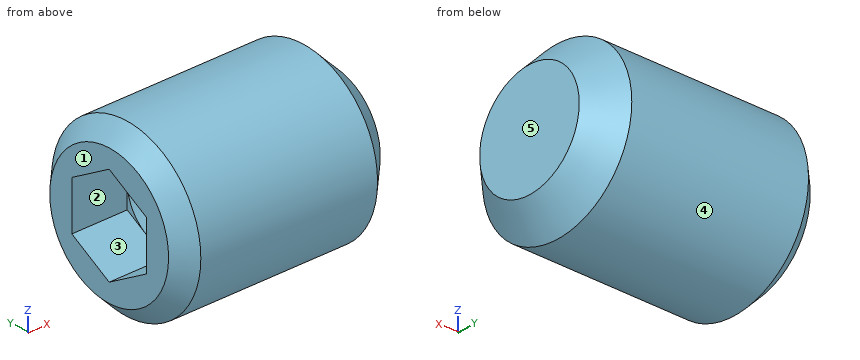
Autodesk Inventor part; units mm, degrees
ref_plane "CP_XY" through (0, 0, 0) normal (1, 0, 0) x (0, 0, -1)
ref_plane "CP_YZ" through (0, 0, 0) normal (0, 0, -1) x (0, 1, 0)
ref_plane "CP_ZX" through (0, 0, 0) normal (0, 1, 0) x (1, 0, 0)
sketch "Sketch_1" plane through (0, 0, 0) normal (0, 0, 1) x (1, 0, 0)
  line L0 (0, 0) -> (-8, 0)
  line L1 (-8, 0) -> (-8, 2.3865)
  line L2 (-8, 2.3865) -> (-7.3865, 3)
  line L3 (-7.3865, 3) -> (-1, 3)
  line L4 (-1, 3) -> (0, 2)
  line L5 (0, 2) -> (0, 0)
  line L6 (0, 0) -> (-8, 0)
revolve "Revolution1" add sketch "Sketch_1" angle 360 about axis through (0, 0, 0) along (1, 0, 0)
thread "Thread1"
sketch "Sketch_2" plane through (-8, 0, 0) normal (-1, 0, 0) x (0, 1, 0)
  line L0 (-1.5, -0.866) -> (0, -1.7321)
  line L1 (0, -1.7321) -> (1.5, -0.866)
  line L2 (1.5, -0.866) -> (1.5, 0.866)
  line L3 (1.5, 0.866) -> (0, 1.7321)
  line L4 (0, 1.7321) -> (-1.5, 0.866)
  line L5 (-1.5, 0.866) -> (-1.5, -0.866)
extrude "Extrusion1" cut sketch "Sketch_2" against normal blind 2
sketch "Sketch_3" plane through (0, 0, 0) normal (0, 0, 1) x (1, 0, 0)
  line L0 (-5.134, 0) -> (-6, 0)
  line L1 (-6, 0) -> (-6, 1.5)
  line L2 (-6, 1.5) -> (-5.134, 0)
  line L3 (-5.134, 0) -> (-6, 0)
revolve "Revolution2" cut sketch "Sketch_3" angle 360 about axis through (-5.134, 0, 0) along (1, 0, 0)
ref_plane "CP_XY" through (0, 0, 0) normal (1, 0, 0) x (0, 0, -1)
ref_plane "CP_YZ" through (0, 0, 0) normal (0, 0, -1) x (0, 1, 0)
ref_plane "CP_ZX" through (0, 0, 0) normal (0, 1, 0) x (1, 0, 0)
properties part number "SET-SCREW6-8"
Source: CAD feature listing. Evaluate the final solid. Frame: model axes, mm. Face numbers are marked on the shaded views. A direction names the side the tool comes from. Round coordinates to 2 decimals unless told otherwise and drop trailing zeros. Write each loop counter-clockwise with the first axis right and the second up, starting at its lowest first coordinate (ties: lowest second). Pieces come first, ordered by that corner, then holes. Notation, with made-up numbers: M -2.5,-10 L 27.5,-10 A15 ccw 27.5,-5 Z; hole C 34,34.5 d4. An arc over 180 degrees is marked long. One line per item, written item: value. Start each with the question number.
Item 1: Section query B-B (x = -1.25). Return the cut outline in (y, z), plus the area to 3 significant figures.
Item 2: Pin query (flat end, axial travel): pin 1 (0.9 mm diameter, centred on y = 0, z = -1, fed in from -X); pin 2 (1 mm diameter, centred on x = -2.5, z = 2, fed in from -Y); pin 3 (0.5 mm diameter, centred on x = -6.5, z = -0.5, fed in from +Y). Return the tip coordinate at first contact, or that it passes through.
Item 3: Mould query, pull axis Z, two halves, no side actions, for the marked faces 3, 4 and 5. Classes: pulls with the +Z half, pulls with the -Z half, needs draft (parallel to the pull), parting line crosses it, or undercut.
Item 4: Section query C-C (x = -5.5). Return the cut outline in (y, z).
Item 5: Set-up query: the marked faces 1 and 2. Return all of +Z, -Z, +X, -X, +Y, -Y with unobstructed straight access to the full face (end or side cutting, diameter ignored); none if empty.
Item 6: Ray query, L1, parallel to Z at x = -7.5, y = -1.3; L2, parallel to Y at x = -1.25, z = -2.45; L3, parallel to Y at x = -6, z = -1.75. Return the intervals inside material, ascending. Write a range as from..to.
Item 7: Section query A-A (x = -7.5). Return the cut outline in (y, z), plus the area to 3 significant figures.
Result set:
1. outline: C 0,0 d6
1. area: 28.3 mm²
2. pin 1: stops at x = -5.97
2. pin 2: stops at y = -2.6
2. pin 3: stops at y = 2.99
3. face 3: undercut
3. face 4: parting line crosses it
3. face 5: needs draft
4. outline: C 0,0 d6; hole C 0,0 d1.27
5. face 1: +Z, -Z, -X, +Y, -Y
5. face 2: -X
6. L1: z = -2.58..-0.98, 0.98..2.58
6. L2: y = -1.73..1.73
6. L3: y = -2.44..2.44
7. outline: C 0,0 d5.77; hole M -1.5,-0.87 L 0,-1.73 L 1.5,-0.87 L 1.5,0.87 L 0,1.73 L -1.5,0.87 Z
7. area: 18.4 mm²
